Input: part model. Units: mm. Frame: model coordinates. A direction names the side the tool comes from. Give positions to 0.01 mm unless a question says otherwise; leave off trailing zeros. Order: outer loops, then holes, each group sorted by start corner. A loop starts at its lowest first (then second) coordinate and runs counter-clockwise, first axis right, second up. Notation, with made-up numbers: M 29.25,77 L 60.25,77 A15 ccw 60.25,100 Z; hole C 12,82.5 d3. An arc over 180 degrees is marked long. Use a Markdown table: item, result.
from build123d import *

# Parameters (mm, degrees)
PAD009_DEPTH    = 2.8
FILLET004_R     = 0.4
SKETCH025_W     = 12.7
SKETCH025_H     = 1.6
POCKET014_DEPTH = 2.801
SKETCH026_R     = 0.25
POCKET015_DEPTH = 2.801
SKETCH028_R     = 8.5
POCKET017_DEPTH = 2.801


with BuildPart() as part:
    # Sketch009 (on Face6 of ShapeBinder008) → Pad009 (new body)
    with BuildSketch(Plane.XZ.offset(60.388718)):
        with BuildLine():
            Line((37.8, 3.127675), (37.8, 0.327675))
            Line((37.8, 0.327675), (23.8, 0.327675))
            ThreePointArc((23.8, 0.327675), (23.4, -0.072325), (23.8, -0.472325))
            Line((23.8, -0.472325), (37.8, -0.472325))
            Line((37.8, -0.472325), (37.8, -33.872325))
            Line((37.8, -33.872325), (23.8, -33.872325))
            ThreePointArc((23.8, -33.872325), (23.4, -34.272325), (23.8, -34.672325))
            Line((23.8, -34.672325), (37.8, -34.672325))
            Line((37.8, -34.672325), (37.8, -37.472325))
            Line((37.8, -37.472325), (35.8, -38.222325))
            Line((35.8, -38.222325), (35.8, -37.472325))
            Line((35.8, -37.472325), (33, -37.472325))
            Line((33, -37.472325), (33, -39.472325))
            Line((33, -39.472325), (25.535898, -37.472325))
            Line((25.535898, -37.472325), (-25.535898, -37.472325))
            Line((-25.535898, -37.472325), (-33, -39.472325))
            Line((-33, -39.472325), (-33, -37.472325))
            Line((-33, -37.472325), (-35.8, -37.472325))
            Line((-35.8, -38.222325), (-35.8, -37.472325))
            Line((-37.8, -37.472325), (-35.8, -38.222325))
            Line((-37.8, -37.472325), (-37.8, -34.672325))
            Line((-37.8, -34.672325), (-23.8, -34.672325))
            ThreePointArc((-23.8, -34.672325), (-23.4, -34.272325), (-23.8, -33.872325))
            Line((-23.8, -33.872325), (-37.8, -33.872325))
            Line((-37.8, -33.872325), (-37.8, -0.472325))
            Line((-37.8, -0.472325), (-23.8, -0.472325))
            ThreePointArc((-23.8, -0.472325), (-23.4, -0.072325), (-23.8, 0.327675))
            Line((-23.8, 0.327675), (-37.8, 0.327675))
            Line((-37.8, 0.327675), (-37.8, 3.127675))
            Line((-37.8, 3.127675), (-35.8, 3.877675))
            Line((-35.8, 3.877675), (-35.8, 3.127675))
            Line((-35.8, 3.127675), (-33, 3.127675))
            Line((-33, 3.127675), (-33, 5.127675))
            Line((-33, 5.127675), (-25.535898, 3.127675))
            Line((-25.535898, 3.127675), (25.535898, 3.127675))
            Line((25.535898, 3.127675), (33, 5.127675))
            Line((33, 5.127675), (33, 3.127675))
            Line((33, 3.127675), (35.8, 3.127675))
            Line((35.8, 3.877675), (35.8, 3.127675))
            Line((37.8, 3.127675), (35.8, 3.877675))
        make_face()
    extrude(amount=-PAD009_DEPTH)

    # Fillet004
    fillet004_edges = [part.edges().sort_by_distance(p)[0] for p in [
        (33, -58.988718, 5.127675),
        (37.8, -58.988718, 3.127675),
        (37.8, -58.988718, 0.327675),
        (37.8, -58.988718, -0.472325),
        (37.8, -58.988718, -33.872325),
        (37.8, -58.988718, -34.672325),
        (37.8, -58.988718, -37.472325),
        (33, -58.988718, -39.472325),
        (-37.8, -58.988718, -33.872325),
        (-37.8, -58.988718, -34.672325),
        (-37.8, -58.988718, -37.472325),
        (-33, -58.988718, -39.472325),
        (-33, -58.988718, 5.127675),
        (-37.8, -58.988718, 3.127675),
        (-37.8, -58.988718, 0.327675),
        (-37.8, -58.988718, -0.472325),
    ]]
    fillet(fillet004_edges, radius=FILLET004_R)

    # Sketch025 (on Face2 of Fillet004) → Pocket014 (cut, through all)
    with BuildSketch(Plane.XZ.offset(60.388718)):
        with Locations((-19.05, -5.2)):
            Rectangle(SKETCH025_W, SKETCH025_H)
        with Locations((19.05, -5.2)):
            Rectangle(SKETCH025_W, SKETCH025_H)
    extrude(amount=-POCKET014_DEPTH, mode=Mode.SUBTRACT)

    # Sketch026 (on Face2 of Pocket014) → Pocket015 (cut, through all)
    with BuildSketch(Plane.XZ.offset(60.388718)):
        with Locations((-25.4, -4.4)):
            Circle(SKETCH026_R)
        with Locations((-12.7, -4.4)):
            Circle(SKETCH026_R)
        with Locations((-12.7, -6)):
            Circle(SKETCH026_R)
        with Locations((-25.4, -6)):
            Circle(SKETCH026_R)
        with Locations((12.7, -4.4)):
            Circle(SKETCH026_R)
        with Locations((12.7, -6)):
            Circle(SKETCH026_R)
        with Locations((25.4, -4.4)):
            Circle(SKETCH026_R)
        with Locations((25.4, -6)):
            Circle(SKETCH026_R)
    extrude(amount=-POCKET015_DEPTH, mode=Mode.SUBTRACT)

    # Sketch028 (on Face2 of Pocket015) → Pocket017 (cut, through all)
    with BuildSketch(Plane.XZ.offset(60.388718)):
        with Locations((-12.8, -24.1)):
            Circle(SKETCH028_R)
        with Locations((12.8, -24.1)):
            Circle(SKETCH028_R)
        with BuildLine():
            ThreePointArc((-2.85, -29.7), (-5.35, -32.2), (-2.85, -34.7))
            Line((-2.85, -34.7), (2.85, -34.7))
            ThreePointArc((2.85, -34.7), (5.35, -32.2), (2.85, -29.7))
            Line((-2.85, -29.7), (2.85, -29.7))
        make_face()
    extrude(amount=-POCKET017_DEPTH, mode=Mode.SUBTRACT)


solid = part.part
1) Cut plane D-D on y = -58.75. State how many separate pieces and enclosed holes the cut face has, and give its area (3 significant figures).
Response values:
| item | result |
|---|---|
| separate pieces | 1 |
| enclosed holes | 5 |
| area | 2,510 mm² |
2) Material intervals for line 1 (X direction, y = -58.3, z = -21); line 2 (Z direction, x = 3, y = -60.2); line 3 (X direction, y = -59.2, z = -19), sorted ascending. Write a range as from..to.
Response values:
| item | result |
|---|---|
| line 1 | x = -37.8..-20.71, -4.89..4.89, 20.71..37.8 |
| line 2 | z = -37.47..-34.7, -29.7..3.13 |
| line 3 | x = -37.8..-19.6, -6..6, 19.6..37.8 |
3) Cut plane A-A on z = -24.1. Return loops of the section in (x, y).
Response values:
| item | result |
|---|---|
| outline | M -37.8,-60.39 L -21.3,-60.39 L -21.3,-57.59 L -37.8,-57.59 Z; M -4.3,-60.39 L 4.3,-60.39 L 4.3,-57.59 L -4.3,-57.59 Z; M 21.3,-60.39 L 37.8,-60.39 L 37.8,-57.59 L 21.3,-57.59 Z |
4) First-contact query: pin 1 Ø1.4 at (x, y) = (-6, -58.5) entering from -Z; pin 2 Ø0.8 at (x, y) = (34, -59) entering from +Z. Flat tips, straight axial feed; report the tip coordinate or a pass-through.
Response values:
| item | result |
|---|---|
| pin 1 | stops at z = -37.47 |
| pin 2 | stops at z = 3.13 |
5) Mould query, pull axis X, two halves, no side actions, for faces 1 (the face through (-31, -59, -0.472)), 2 (the face through (29.065, -59.008, -38.418)), 3 (the face through (-37.8, -59, 2)), 4 (the face through (0, -59, -34.7)). Classes: released by +X, released by -X, zero draft, split by the parting line, or undercut.
Response values:
| item | result |
|---|---|
| face 1 | zero draft |
| face 2 | undercut |
| face 3 | released by -X |
| face 4 | undercut |
6) Cut plane B-B on x = -10. Return loops of the section in (y, z).
Response values:
| item | result |
|---|---|
| outline | M -60.39,-37.47 L -57.59,-37.47 L -57.59,-32.13 L -60.39,-32.13 Z; M -60.39,-16.07 L -57.59,-16.07 L -57.59,3.13 L -60.39,3.13 Z |
7) Cut plane C-C on z = -31. Return loops of the section in (x, y), and give its area (3 significant figures).
Response values:
| item | result |
|---|---|
| outline | M -37.8,-60.39 L -17.76,-60.39 L -17.76,-57.59 L -37.8,-57.59 Z; M -7.84,-60.39 L -5.04,-60.39 L -5.04,-57.59 L -7.84,-57.59 Z; M 5.04,-60.39 L 7.84,-60.39 L 7.84,-57.59 L 5.04,-57.59 Z; M 17.76,-60.39 L 37.8,-60.39 L 37.8,-57.59 L 17.76,-57.59 Z |
| area | 128 mm² |
8) Reachability of faces 5 (the face through (0, -59, -29.7)), 6 (the face through (-31, -59, 0.328)), 7 (the face through (33, -59, -38)), 8 (the face through (31, -59, -33.872)), 9 (the face through (34, -59, 3.128)) from +Z, -Z, +X, -X, +Y, -Y: full face, straight path, thin tool, end or side. Return the list, or none.
Response values:
| item | result |
|---|---|
| face 5 | +Y, -Y |
| face 6 | -X, +Y, -Y |
| face 7 | -Z, +Y, -Y |
| face 8 | +X, +Y, -Y |
| face 9 | +Z, +Y, -Y |
